Could you check a few things on this model? Use its own coordinates, in mm. A direction names the side the tool comes from. Coordinates: 2 decimals unless noted, no trailing zeros. Loops run counter-clockwise (first coordinate to the right, second up) from the corner with the lowest first, then second, coordinate; pieces in that order, holes last.
from build123d import *

# Parameters (mm, degrees)
F0_W     = 5
F0_H     = 5
F2_DEPTH = 136.5
F1_R     = 2.5
F3_DEPTH = 30


with BuildPart() as f2:
    # F0 (on Top) → F2 (new body)
    with BuildSketch(Plane.XY):
        with Locations((-0.112459, -0.150917)):
            Rectangle(F0_W, F0_H)
    extrude(amount=F2_DEPTH)

    # F1 (on Top) → F3 (join)
    with BuildSketch(Plane.XY):
        with Locations((-0.112376, -0.150785)):
            Circle(F1_R)
    extrude(amount=-F3_DEPTH)


solid = f2.part
(1) Which directions (+Z, -Z, +X, -X, +Y, -Y) give clear straight access to the entire face, cutting with the end or side of a thin tool? Please do faces 4 (the face through (0, -2.651, 67)), 5 (the face through (-2.1, -1.67, -14.79)).
Answers:
face 4: +Z, -Z, +X, -X, -Y
face 5: -Z
(2) We'd pull the mould along Z, two halves only. Please class faces 1 (the face through (-2.2, -1.8, 0)), 2 (the face through (0, 2.349, 67)), 3 (the face through (0, 0, 136.5)): +Z half, -Z half, draft (parallel to the pull), parting line (faces both ways), or undercut.
Answers:
face 1: -Z half
face 2: draft
face 3: +Z half
(3) I need wall thicknesses on probe 1 along Z at (x, y) = (-2.2, 1.9); probe 2 along X at (y, z) = (0.5, -15.5); probe 3 along X at (y, z) = (1.5, -15.5). Which ranges of each line are inside material? Lowest first, please.
Answers:
probe 1: z = 0 to 136.5
probe 2: x = -2.53 to 2.3
probe 3: x = -1.99 to 1.77
(4) Imagine slicing it at A-A, the plane y = 0.9. Write out the boundary of the cut face in (x, z).
Answers:
outline: (-2.61, 0) - (-2.38, 0) - (-2.38, -30) - (2.16, -30) - (2.16, 0) - (2.39, 0) - (2.39, 136.5) - (-2.61, 136.5) - close
